Input: part model. Units: mm. Frame: model coordinates. A direction names the side the tool comes from. Coordinates: 2 decimals unless noted, no trailing zeros. Loops run counter-clockwise (first coordinate to the right, second up) from the corner with the lowest first, then second, coordinate; pieces in that order, holes last.
```python
from build123d import *

# Parameters (mm, degrees)
SKETCH1_R           = 1
SKETCH1_R_2         = 1.5
BOSS_EXTRUDE1_DEPTH = 3


with BuildPart() as part:
    # Sketch1 → Boss-Extrude1 (new body)
    with BuildSketch(Plane.XY):
        with BuildLine():
            Line((5.6, -29.5), (-5.6, -29.5))
            ThreePointArc((-5.6, -29.5), (-5.953553391, -29.646446609), (-6.1, -30))
            Line((-6.1, -30), (-6.1, -32))
            ThreePointArc((-6.1, -32), (-6.246446609, -32.353553391), (-6.6, -32.5))
            Line((-6.6, -32.5), (-9.6, -32.5))
            ThreePointArc((-9.6, -32.5), (-9.953553391, -32.353553391), (-10.1, -32))
            Line((-10.1, -32), (-10.1, -22.5))
            Line((-10.1, -22.5), (-10.1, 22.5))
            Line((-10.1, 22.5), (-10.1, 32))
            ThreePointArc((-10.1, 32), (-9.953553391, 32.353553391), (-9.6, 32.5))
            Line((-9.6, 32.5), (-6.6, 32.5))
            ThreePointArc((-6.6, 32.5), (-6.246446609, 32.353553391), (-6.1, 32))
            Line((-6.1, 32), (-6.1, 30))
            ThreePointArc((-6.1, 30), (-5.953553391, 29.646446609), (-5.6, 29.5))
            Line((-5.6, 29.5), (5.6, 29.5))
            ThreePointArc((5.6, 29.5), (5.953553391, 29.646446609), (6.1, 30))
            Line((6.1, 30), (6.1, 32))
            ThreePointArc((6.1, 32), (6.246446609, 32.353553391), (6.6, 32.5))
            Line((6.6, 32.5), (9.6, 32.5))
            ThreePointArc((9.6, 32.5), (9.953553391, 32.353553391), (10.1, 32))
            Line((10.1, 32), (10.1, 22.5))
            Line((10.1, 22.5), (10.1, -22.5))
            Line((10.1, -22.5), (10.1, -32))
            ThreePointArc((10.1, -32), (9.953553391, -32.353553391), (9.6, -32.5))
            Line((9.6, -32.5), (6.6, -32.5))
            ThreePointArc((6.6, -32.5), (6.246446609, -32.353553391), (6.1, -32))
            Line((6.1, -32), (6.1, -30))
            ThreePointArc((6.1, -30), (5.953553391, -29.646446609), (5.6, -29.5))
        make_face()
        with Locations((0, 13.9)):
            Circle(SKETCH1_R, mode=Mode.SUBTRACT)
        with Locations(Location((0, -13.9, 0), (0, 0, 180))):
            Circle(SKETCH1_R, mode=Mode.SUBTRACT)
        with Locations((0, 24.85)):
            Circle(SKETCH1_R_2, mode=Mode.SUBTRACT)
        with BuildLine():
            Line((5.25, -11.25), (-5.25, -11.25))
            ThreePointArc((-5.25, -11.25), (-5.851040764, -11.001040764), (-6.1, -10.4))
            Line((-6.1, -10.4), (-6.1, 10.4))
            ThreePointArc((-6.1, 10.4), (-5.851040764, 11.001040764), (-5.25, 11.25))
            Line((-5.25, 11.25), (5.25, 11.25))
            ThreePointArc((5.25, 11.25), (5.851040764, 11.001040764), (6.1, 10.4))
            Line((6.1, 10.4), (6.1, -10.4))
            ThreePointArc((6.1, -10.4), (5.851040764, -11.001040764), (5.25, -11.25))
        make_face(mode=Mode.SUBTRACT)
    extrude(amount=BOSS_EXTRUDE1_DEPTH)


solid = part.part
```
Item 1: Reachability of faces 4 (the face through (0, 11.25, 1)), 5 (the face through (6.1, -31, 1)), 6 (the face through (-7, 0, 0)), 7 (the face through (6.1, 31, 1)) from +Z, -Z, +X, -X, +Y, -Y: full face, straight path, thin tool, end or side. Return the list, or none.
Result:
face 4: +Z, -Z
face 5: +Z, -Z, -Y
face 6: -Z, +X, -X, +Y, -Y
face 7: +Z, -Z, +Y
Item 2: Section query B-B (y = -13.9). Output: boundary loops of the cut face in (x, z), then the cut area to 3 significant figures.
Result:
outline: (-10.1, 0) - (-1, 0) - (-1, 3) - (-10.1, 3) - close; (1, 0) - (10.1, 0) - (10.1, 3) - (1, 3) - close
area: 54.6 mm2
Item 3: Section query D-D (z = 1.05). Count the separate pieces of the cut face and the enclosed holes in it, then the cut area to 3 significant figures.
Result:
separate pieces: 1
enclosed holes: 4
area: 952 mm2
Item 4: Contact query for flat-ended pins moving along their axis: P1, Ø0.9, axis at x = -0.5, z = 1.5, coming from the -Y side; P2, Ø1.6, axis at x = 0, y = 13.9, coming from the -Z side. Output: stop coordinate, or through.
Result:
P1: stops at y = -29.5
P2: passes through
Item 5: Section query A-A (x = 2.5). Output: boundary loops of the cut face in (y, z), then the cut area to 4 significant figures.
Result:
outline: (-29.5, 0) - (-11.25, 0) - (-11.25, 3) - (-29.5, 3) - close; (11.25, 0) - (29.5, 0) - (29.5, 3) - (11.25, 3) - close
area: 109.5 mm2
Item 6: Section query C-C (x = 0). Output: boundary loops of the cut face in (y, z).
Result:
outline: (-29.5, 0) - (-14.9, 0) - (-14.9, 3) - (-29.5, 3) - close; (-12.9, 0) - (-11.25, 0) - (-11.25, 3) - (-12.9, 3) - close; (11.25, 0) - (12.9, 0) - (12.9, 3) - (11.25, 3) - close; (14.9, 0) - (23.35, 0) - (23.35, 3) - (14.9, 3) - close; (26.35, 0) - (29.5, 0) - (29.5, 3) - (26.35, 3) - close
Item 7: Mould query, pull axis Y, two halves, no side actions, for faces 1 (the face through (0, -11.25, 1)), 2 (the face through (-10.1, 0, 1)), 3 (the face through (-8, -32.5, 1)). Classes: +Y half, -Y half, draft (parallel to the pull), parting line (faces both ways), or undercut.
Result:
face 1: undercut
face 2: draft
face 3: -Y half
Item 8: Line query: L1, parallel to Y at x = 0, z = 1.3; L2, parallel to Y at x = 2.5, z = 0.75; L3, parallel to X at y = 9, z = 0.2. Output: solid intervals per line, ascending.
Result:
L1: y = -29.5 to -14.9, -12.9 to -11.25, 11.25 to 12.9, 14.9 to 23.35, 26.35 to 29.5
L2: y = -29.5 to -11.25, 11.25 to 29.5
L3: x = -10.1 to -6.1, 6.1 to 10.1
